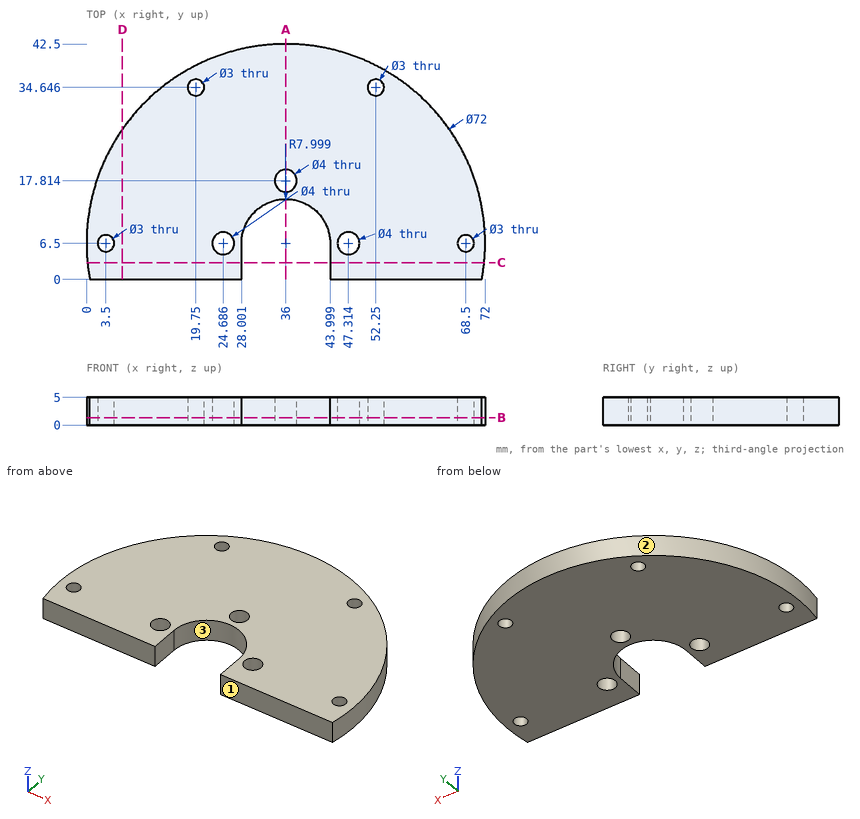
Design review of the part shown in the three views and the two pictorial views. Dimensions are in mm from the part's minimum x, y and z. Give positions to 0.01 mm unless a question says otherwise; leave off trailing zeros. Loops run counter-clockwise (first coordinate to the right, second up) from the corner with the lowest first, then second, coordinate; pieces in that order, holes last. Notation, with made-up numbers: (5.5, 9.25) -> (21.5, 9.25) arc R18 ccw to (21.5, 30.25) -> close; hole circle Ø10 at (45, -19.75). An arc over 180 degrees is marked (long way). Write each question's results on one line, items separated by ' | '.
1) Take a section at C-C, the plane y = 3. Give the boundary of the cut face in (x, z).
Conclusion:
outline: (0.17, 0) -> (28, 0) -> (28, 5) -> (0.17, 5) -> close; (44, 0) -> (71.83, 0) -> (71.83, 5) -> (44, 5) -> close
2) Take a section at B-B, the plane z = 1.35. Give the boundary of the cut face in (x, y).
Conclusion:
outline: (0.59, 0) -> (28, 0) -> (28, 6.5) arc R8 cw to (44, 6.5) -> (44, 0) -> (71.41, 0) arc R36 ccw (long way) to start; hole circle Ø3 at (3.5, 6.5); hole circle Ø3 at (19.75, 34.65); hole circle Ø4 at (24.69, 6.5); hole circle Ø4 at (36, 17.81); hole circle Ø4 at (47.31, 6.5); hole circle Ø3 at (52.25, 34.65); hole circle Ø3 at (68.5, 6.5)
3) Draft analysis for pull direction X (two halves, no side actions). For the marked faces 1, 2 and 3, state which applies: pulls with the +X half, pulls with the -X half, needs draft (parallel to the pull), parting line crosses it, or undercut.
Conclusion:
face 1: needs draft | face 2: parting line crosses it | face 3: undercut
4) Insertion check: pin 1 Ø3 at (x, y) = (47.31, 6.5) entering from -Z; pin 2 Ø1 at (y, z) = (17.5, 2.5) entering from +X (1 decimal); pin 3 Ø12 at (x, y) = (26, 29.5) entering from -Z; pin 4 Ø1.5 at (y, z) = (25, 3.5) entering from -X. Each pin has a flat end and moves straight along its axis. Give the tip position at first contact, or say it passes through.
Conclusion:
pin 1: passes through | pin 2: stops at x = 70.4 | pin 3: stops at z = 0 | pin 4: stops at x = 4.68
5) Take a section at A-A, the plane x = 36. Give the boundary of the cut face in (y, z), plus the area to 3 significant figures.
Conclusion:
outline: (14.5, 0) -> (15.81, 0) -> (15.81, 5) -> (14.5, 5) -> close; (19.81, 0) -> (42.5, 0) -> (42.5, 5) -> (19.81, 5) -> close | area: 120 mm^2
6) Take a section at D-D, the plane x = 6.5. Give the boundary of the cut face in (y, z).
Conclusion:
outline: (0, 0) -> (27.13, 0) -> (27.13, 5) -> (0, 5) -> close
7) For line 1 along Y through (x, z) = (36, 1.15); line 2 along Y through (x, z) = (68.5, 1.75) (1 decimal); line 3 along X through (y, z) = (17, 0.35) (1 decimal), list the stretches that pass through material, from the lowest coordinate up. Write a range as from..to.
Conclusion:
line 1: y = 14.5..15.81, 19.81..42.5 | line 2: y = 0..5, 8..22 | line 3: x = 1.6..34.2, 37.8..70.4
